Design review of the part built by this model. Coordinates are the model's own, in mm. Round coordinates to 2 decimals unless told otherwise and drop trailing zeros. Write each loop counter-clockwise with the first axis right and the second up, starting at its lowest first coordinate (ties: lowest second). Pieces come first, ordered by that corner, then holes.
from build123d import *

# Parameters (mm, degrees)
F0_W           = 236.5375
F0_H           = 123.825
F1_DEPTH       = 2.032
F2_R           = 6.35
F3_D           = 4.9149
F5_D           = 4.9149
F5_CSINK_D     = 8.89
F5_CSINK_ANGLE = 100
F6_D           = 4.9149


with BuildPart() as f1:
    # F0 (on Top) → F1 (new body)
    with BuildSketch(Plane.XY):
        Rectangle(F0_W, F0_H)
    extrude(amount=F1_DEPTH)

    # F2
    f2_edges = [f1.edges().sort_by_distance(p)[0] for p in [
        (118.26875, -61.9125, 1.016),
        (118.26875, 61.9125, 1.016),
        (-118.26875, -61.9125, 1.016),
        (-118.26875, 61.9125, 1.016),
    ]]
    fillet(f2_edges, radius=F2_R)

    # F3 (through all)
    with Locations(Plane(origin=(0, 0, 0), x_dir=(1, 0, 0), z_dir=(0, 0, -1))):
        with Locations((-107.95, -47.625), (-107.95, 47.625), (80.16875, 47.625), (80.16875, -47.625)):
            Hole(F3_D / 2)

    # F5 (through all)
    with Locations(Plane.XY.offset(2.032)):
        with Locations((-77.7875, 48.41875), (-77.7875, -48.41875)):
            CounterSinkHole(F5_D / 2, F5_CSINK_D / 2, counter_sink_angle=F5_CSINK_ANGLE)

    # F6 (through all)
    with Locations(Plane.XY.offset(2.032)):
        with Locations((107.95, 48.41875), (107.95, -48.41875)):
            Hole(F6_D / 2)


solid = f1.part
1) For line 1 along Y through (x, z) = (107.95, 0.45); line 2 along Y through (x, z) = (-107.95, 0.9); line 3 along X through (y, z) = (-57, 1.9), list the stretches that pass through material, from the lowest coordinate up.
2) Add section A-A on x = 107.95. State the section outline as (y, z) points, and give its area (3 significant figures).
3) For P1, Ø4, axis at x = -107.95, y = 47.625, coming from the +Z side; P2, Ø5.5, axis at x = -77.79, y = 48.42, coming from the +Z side, all flat-tipped, find the tip position at first contact; note any pin that passes through.
4) The part is to be moulded in two halves that separate along X. For faces 1 (the face through (116.36, -60.1, 1.03)), 2 (the face through (-116.46, 60, 1.03)), 3 (the face through (110.405, -48.311, 1.002)), 4 (the face through (-2, 1, 2.032)), say which applies: pulls with the +X half, pulls with the -X half, needs draft (parallel to the pull), parting line crosses it, or undercut.
Computed:
1. line 1: y = -61.91 to -50.88, -45.96 to 45.96, 50.88 to 61.91
1. line 2: y = -61.91 to -50.08, -45.17 to 45.17, 50.08 to 61.91
1. line 3: x = -118.1 to 118.1
2. outline: (-61.91, 0) - (-50.88, 0) - (-50.88, 2.03) - (-61.91, 2.03) - close; (-45.96, 0) - (45.96, 0) - (45.96, 2.03) - (-45.96, 2.03) - close; (50.88, 0) - (61.91, 0) - (61.91, 2.03) - (50.88, 2.03) - close
2. area: 232 mm2
3. P1: passes through
3. P2: stops at z = 0.61
4. face 1: pulls with the +X half
4. face 2: pulls with the -X half
4. face 3: undercut
4. face 4: needs draft
